Here's how the part is built. I have some questions about the finished solid (model axes, mm). Face numbers are marked on the shaded views. A direction names the side the tool comes from. Coordinates: 2 decimals unless noted, no trailing zeros. Order: outer loops, then holes, each group sorted by start corner. A loop starts at its lowest first (then second) coordinate and runs counter-clockwise, first axis right, second up. Notation, with made-up numbers: M 43,27.5 L 73,27.5 A25 cw 73,43.5 Z; hole C 56,-17.5 d7. An arc over 180 degrees is marked long. One line per question, with ' | ' between items. Start each with the question number.
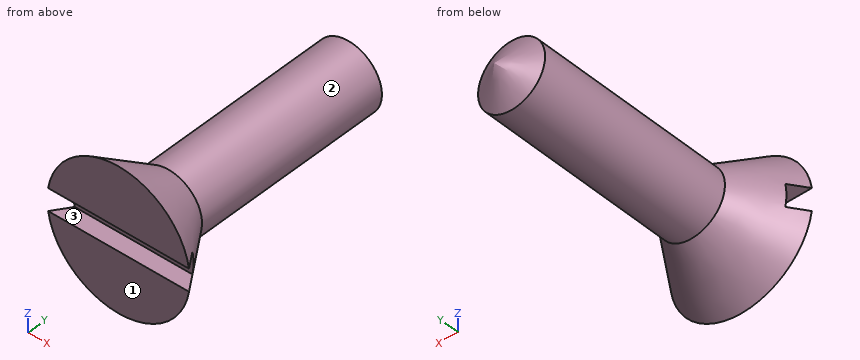
Autodesk Inventor part; units mm, degrees
ref_plane "Work Plane1" through (0, 5, 0) normal (0, 1, 0) x (-1, 0, 0)
ref_plane "Work Plane2" through (0, 24.732, 0) normal (0, 1, 0) x (1, 0, 0)
ref_plane "YZ Plane" through (0, 0, 0) normal (1, 0, 0) x (0, 1, 0)
sketch "Sketch1" plane through (0, 0, 0) normal (0, 1, 0) x (-1, 0, 0)
  circle A0 centre (0, 0) radius 6.385
  dimension "d0" = 12.77
ref_plane "Work Plane1" through (0, 5, 0) normal (0, 1, 0) x (-1, 0, 0)
sketch "Sketch2" plane through (0, 5, 0) normal (0, 1, 0) x (-1, 0, 0)
  circle A0 centre (0, 0) radius 3
  dimension "d2" = 6
extrude "Extrusion1" add sketch "Sketch2" along normal blind 18
loft "Loft1" add profiles "Sketch1" section 2 edges at (3, 5, 0)
sketch "Sketch3" plane through (0, 0, 0) normal (1, 0, 0) x (0, 1, 0)
  line L0 (1.5, 1) -> (-1.5, 1)
  line L1 (-1.5, 1) -> (-1.5, -1)
  line L2 (-1.5, -1) -> (1.5, -1)
  line L3 (1.5, -1) -> (1.5, 1)
  line L4 (1.5, 1) -> (-1.5, -1) construction
  line L5 (-1.5, 1) -> (1.5, -1) construction
  point P0 (0, 0)
  dimension "d9" = 3
  dimension "d10" = 2
extrude "Extrusion2" cut sketch "Sketch3" along normal mid plane 15
sketch "Sketch5" plane through (0, 0, 0) normal (1, 0, 0) x (0, 1, 0)
  line L0 (23, -3) -> (23, 3)
  line L1 (23, 3) -> (24.7321, 0)
  line L2 (24.7321, 0) -> (23, -3)
  line L3 (23, -3) -> (23, 3)
  point P0 (0, 0)
  dimension "d13" = 120
sketch "Sketch8" plane through (0, 0, 0) normal (1, 0, 0) x (0, 1, 0)
  point P0 (0, 0)
ref_plane "Work Plane2" through (0, 24.732, 0) normal (0, 1, 0) x (1, 0, 0)
sketch "Sketch9" plane through (0, 24.732, 0) normal (0, 1, 0) x (1, 0, 0)
  circle A0 centre (0, 0) radius 0.0005
  dimension "d15" = 0.001
loft "Loft2" add profiles "Sketch9" section 1 edges at (3, 23, 0)
1. I need wall thicknesses on line 1 (X direction, y = 7.75, z = 1); line 2 (Y direction, x = 3, z = -3.5); line 3 (Z direction, x = -1.75, y = 18.75). Which ranges of each line are inside material? Lowest first, please.
2. Imagine slicing it at A-A (y = 9.5). List the corners of the cut face in (x, z) for me.
3. Will these pins go through, and if not, where does the flat tip stop? pin 1 (6 mm diameter, centred on y = 20.5, z = -2, fed in from -X); pin 2 (6 mm diameter, centred on x = -5, y = 18, fed in from -Z); pin 3 (2 mm diameter, centred on x = 0, y = 9, fed in from -Z); pin 4 (1.5 mm diameter, centred on y = 15, z = 4, fed in from -X).
4. Which directions (+Z, -Z, +X, -X, +Y, -Y) give clear straight access to the entire face, cutting with the end or side of a thin tool? Please do the marked faces 1, 2 and 3.
Entries:
1) line 1: -2.83 to 2.83 | line 2: 0 to 2.62 | line 3: -2.44 to 2.44
2) outline: C 0,0 d6
3) pin 1: x = -3 | pin 2: z = -2.24 | pin 3: z = -3 | pin 4: through
4) face 1: +Z, -Z, +X, -X, -Y | face 2: +Y | face 3: +X, -X, -Y
